Work out the finished part from the listing and answer in its coordinate system (mm). Face numbers are marked on the shaded views. A direction names the side the tool comes from. Coordinates: 2 decimals unless noted, no trailing zeros. Loops run counter-clockwise (first coordinate to the right, second up) from the corner with the lowest first, then second, coordinate; pieces in that order, holes last. Notation, with made-up numbers: M 81.5,67.25 L 113.5,67.25 A17 cw 113.5,96.25 Z; hole C 5.5,49 d2. An arc over 180 degrees is marked long. Write each question's results on one line, items separated by ' | '.
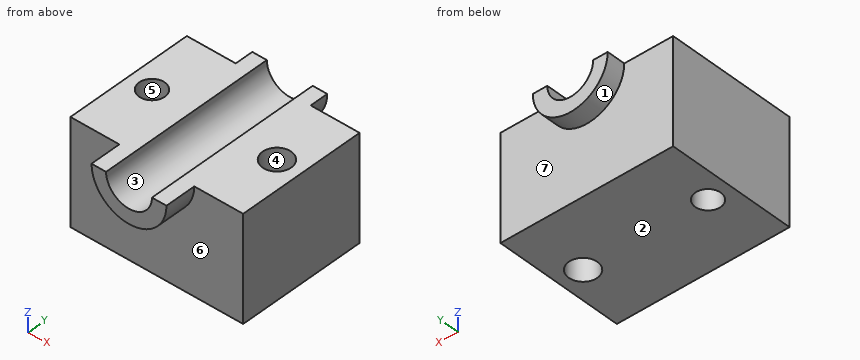
```python
from build123d import *

# Parameters (mm, degrees)
F0_W     = 104.885712266
F0_H     = 78.7287391722
F1_DEPTH = 63.754
F3_DEPTH = 18.796
F4_DEPTH = 105.156
F5_DEPTH = 108.712
F6_R     = 7.7678468682
F6_R_2   = 8.6774880562
F7_DEPTH = 90.17


with BuildPart() as f1:
    # F0 (on Top) → F1 (new body)
    with BuildSketch(Plane.XY):
        with Locations((4.3426826596, 21.0932102054)):
            Rectangle(F0_W, F0_H)
    extrude(amount=F1_DEPTH)

    # F2 (on face) → F3 (join)
    with BuildSketch(Plane.XZ.offset(18.2711593807)):
        with BuildLine():
            Line((-9.586125523, 63.754), (-18.415103221, 63.754))
            ThreePointArc((-18.415103221, 63.754), (4.3426826596, 40.9962141193), (27.1004685403, 63.754))
            Line((27.1004685403, 63.754), (18.2714908423, 63.754))
            ThreePointArc((18.2714908423, 63.754), (4.3426826596, 49.8251918173), (-9.586125523, 63.754))
        make_face()
    extrude(amount=F3_DEPTH)

    # F4 (cut): a face of the model
    f4_faces = [f1.faces().sort_by_distance(p)[0] for p in [
        (4.3426826596, -18.2711593807, 57.8424302036),
    ]]
    extrude(f4_faces, amount=-F4_DEPTH, mode=Mode.SUBTRACT)

    # F5 (add): a face of the model
    f5_faces = [f1.faces().sort_by_distance(p)[0] for p in [
        (22.6859796913, -37.0671593807, 63.2451204375),
    ]]
    extrude(f5_faces, amount=-F5_DEPTH)

    # F6 (on face) → F7 (cut)
    with BuildSketch(Plane.XY.offset(63.754)):
        with Locations((-33.9234930099, 21.0932102054)):
            Circle(F6_R)
        with Locations((41.9430036665, 21.0932102054)):
            Circle(F6_R_2)
    extrude(amount=-F7_DEPTH, mode=Mode.SUBTRACT)


solid = f1.part
```
1) Find section B-B, the plane y = 19. Give the vertices of the cut face in (x, z), and give its area (3 significant figures).
Check result:
outline: M -48.1,0 L -41.4,0 L -41.4,63.75 L -48.1,63.75 Z; M -26.44,0 L 33.52,0 L 33.52,63.75 L 18.27,63.75 A13.93 cw -9.59,63.75 L -26.44,63.75 Z; M 50.36,0 L 56.79,0 L 56.79,63.75 L 50.36,63.75 Z | area: 4,350 mm^2
2) Find section A-A, the plane x = 37.5. Give the vertices of the cut face in (y, z).
Check result:
outline: M -18.27,0 L 13.64,0 L 13.64,63.75 L -18.27,63.75 Z; M 28.55,0 L 60.46,0 L 60.46,63.75 L 28.55,63.75 Z
3) For a pull along X with two mould halves and no side action, classify the marked faces 1, 2, 3 and 4 as released by +X, released by -X, zero draft, split by the parting line, or undercut.
Check result:
face 1: split by the parting line | face 2: zero draft | face 3: undercut | face 4: undercut
4) Which of the six approach directions +Z, -Z, +X, -X, +Y, -Y give full straight-line access (tool end or side, diameter ignored) to the marked faces 5, 6 and 7?
Check result:
face 5: +Z, -Z | face 6: -Z, -Y | face 7: -Z, +Y
5) Find section C-C, the plane z = 32. Give the vertices of the cut face in (x, y).
Check result:
outline: M -48.1,-18.27 L 56.79,-18.27 L 56.79,60.46 L -48.1,60.46 Z; hole C -33.92,21.09 d15.54; hole C 41.94,21.09 d17.35
6) Given pin 1 Ø8 at (y, z) = (-24.5, 52.5) entering from -X; pin 2 Ø5 at (x, z) = (42, 39) entering from -Y, each flat-ended and moving along its own axis, determine where each tip first touches the part or whether it passes through.
Check result:
pin 1: x = -17.23 | pin 2: y = -18.27
7) Straight lines are drawn through the part: probe 1 along X at (y, z) = (21, 7); probe 2 along X at (y, z) = (26.5, 55.5); probe 3 along Y at (x, z) = (44, 53.5). For each, find the intervals that lie inside material, in ascending order. Write a range as [from, to].
Check result:
probe 1: [-48.1, -41.69], [-26.16, 33.27], [50.62, 56.79] | probe 2: [-48.1, -39.5], [-28.35, -6.88], [15.56, 35.16], [48.73, 56.79] | probe 3: [-18.27, 12.66], [29.52, 60.46]
8) Find section D-D, the plane x = -11.5. Give the vertices of the cut face in (y, z).
Check result:
outline: M -37.07,47.42 L -18.27,47.42 L -18.27,0 L 60.46,0 L 60.46,47.42 L 71.64,47.42 L 71.64,63.75 L -37.07,63.75 Z
